from build123d import *


with BuildPart() as f1:
    # F0 (on Front) → F1 (revolve)
    with BuildSketch(Plane.XZ):
        Polygon((8, 49.8), (3, 49.8), (2.555618, 49.211922), (2.555618, 48.211922), (3.537895, 45.965945), (3.537895, 41.892459), (2.05, 39.236551), (2.05, 7.1), (2.05, 0), (2.476728, 0), (3.047144, 0.404497), (3.047144, 4.667719), (2.476728, 5), (2.476728, 7.1), (11.011527, 7.1), (11.011527, 8.032141), (3, 8.032141), (3, 10.032141), (11.011527, 10.032141), (11.011527, 11.032141), (3, 11.032141), (3, 13.232141), (11.011527, 13.232141), (11.011527, 14.232141), (3, 14.232141), (3, 16.432141), (11.011527, 16.432141), (11.011527, 17.432141), (3, 17.432141), (3, 19.532141), (11, 19.532141), (11, 20.532141), (6.5, 20.532141), (6.5, 21.932141), (11, 21.932141), (11, 22.932141), (3, 22.932141), (3, 25.032141), (11, 25.032141), (11, 26.032141), (3, 26.032141), (3, 29.032141), (11, 29.032141), (11, 30.032141), (3, 30.032141), (3, 32.132141), (11, 32.132141), (11, 33.132141), (4.5, 33.132141), (4.5, 34.524906), (8, 34.524906), (8, 35.524906), (4.5, 35.524906), (4.5, 37.1), (8, 37.1), (8, 40.1), (6, 40.1), (6, 46.1), (8, 46.1), align=None)
    revolve(axis=Axis((0, 0, 18.136091), (0, 0, -1)))


solid = f1.part
Design review of the part built by this model. Coordinates are the model's own, in mm. Round coordinates to 2 decimals unless told otherwise and drop trailing zeros. One line per item, written item: value. Start each with the question number.
Q1. The part is to be moulded in two halves that separate along Z. For faces 1 (the face through (-0.4, -3.02, 2.57)), 2 (the face through (-5.158, 3.955, 21.242)), say which applies: pulls with the +Z half, pulls with the -Z half, needs draft (parallel to the pull), parting line crosses it, or undercut.
Q2. To check wall thickness, follow probe 1 along X at (y, z) = (0, 43.3); probe 2 along Y at (x, z) = (0, 18); probe 3 along Y at (x, z) = (0, 48.95). State the ranges of each line that lie inside material, in increasing order.
Q3. Add section A-A (y = 7). State how many separate pieces and enclosed holes the cut face has, then the cut area to 3 significant figures.
Q4. Insertion check: P1, Ø4, axis at x = -5.5, z = 18, coming from the +Y side; P2, Ø3, axis at x = 3, z = 13.5, coming from the +Y side; P3, Ø8, axis at x = -7.5, y = -1.5, coming from the -Z side. Each pin has a flat end and moves straight along its axis. Give the tip position at first contact, or say it passes through.
Response:
1. face 1: needs draft
1. face 2: undercut
2. probe 1: x = -6 to -3.54, 3.54 to 6
2. probe 2: y = -3 to -2.05, 2.05 to 3
2. probe 3: y = -8 to -2.56, 2.56 to 8
3. separate pieces: 12
3. enclosed holes: 0
3. area: 211 mm^2
4. P1: stops at y = 10.41
4. P2: stops at y = 10.91
4. P3: stops at z = 7.1
